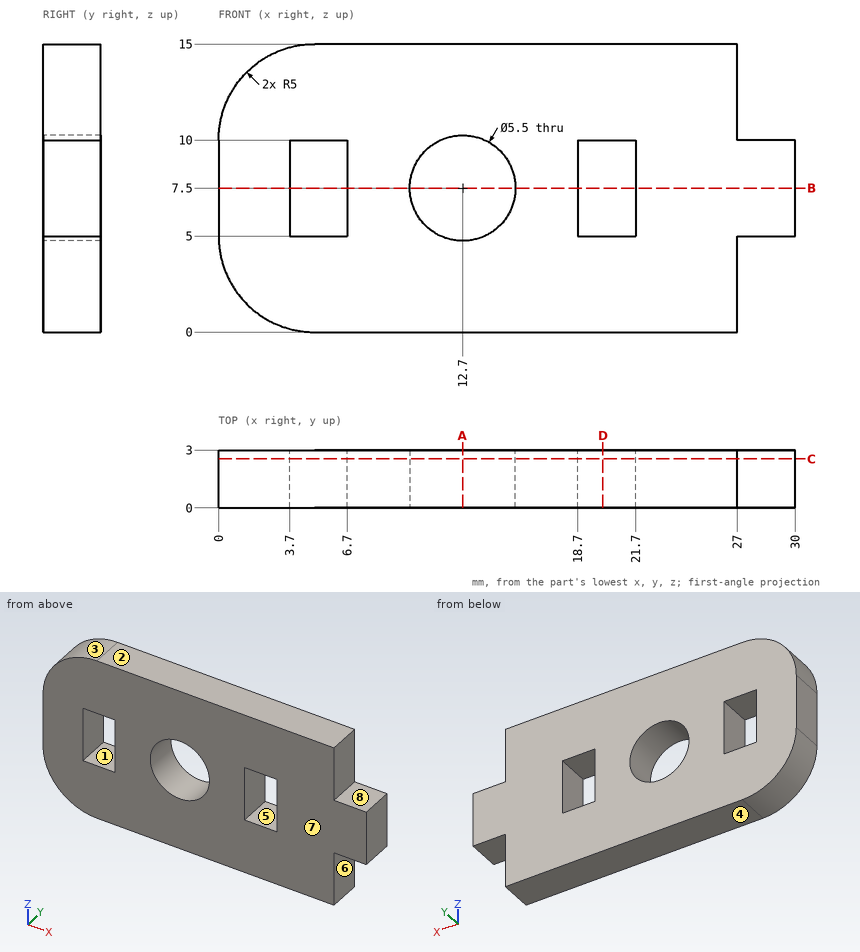
Here's the drawing with two shaded views (mm, measured from the low corner). I have some questions. A direction names the side the tool comes from. Coordinates: 2 decimals unless noted, no trailing zeros. Order: outer loops, then holes, each group sorted by start corner. A loop starts at its lowest first (then second) coordinate and runs counter-clockwise, first axis right, second up. Notation, with made-up numbers: M 25.5,13 L 45.5,13 A29 ccw 45.5,43 Z; hole C -7,81 d6. An arc over 180 degrees is marked long. Answer as CSV lines item,"result".
Item 1: Imagine slicing it at C-C on y = 2.55. Write out the boundary of the cut face in (x, z).
Results found:
outline,"M 0,5 A5 ccw 5,0 L 27,0 L 27,5 L 30,5 L 30,10 L 27,10 L 27,15 L 5,15 A5 ccw 0,10 Z; hole M 3.7,5 L 6.7,5 L 6.7,10 L 3.7,10 Z; hole C 12.7,7.5 d5.5; hole M 18.7,5 L 21.7,5 L 21.7,10 L 18.7,10 Z"
Item 2: Imagine slicing it at B-B on z = 7.5. Write out the boundary of the cut face in (x, y).
Results found:
outline,"M 0,0 L 3.7,0 L 3.7,3 L 0,3 Z; M 6.7,0 L 9.95,0 L 9.95,3 L 6.7,3 Z; M 15.45,0 L 18.7,0 L 18.7,3 L 15.45,3 Z; M 21.7,0 L 30,0 L 30,3 L 21.7,3 Z"
Item 3: Imagine slicing it at D-D on x = 20. Write out the boundary of the cut face in (y, z), plus the area to 3 significant figures.
Results found:
outline,"M 0,0 L 3,0 L 3,5 L 0,5 Z; M 0,10 L 3,10 L 3,15 L 0,15 Z"
area,"30.0 mm2"
Item 4: If I drill on line 1 (X direction, y = 0.9, z = 7.5); line 2 (Z direction, x = 5, y = 2.2); line 3 (X direction, y = 1.9, z = 6.5), over which ranges is the centre line in solid material (lowest first)?
Results found:
line 1,"0 to 3.7, 6.7 to 9.95, 15.45 to 18.7, 21.7 to 30"
line 2,"0 to 5, 10 to 15"
line 3,"0 to 3.7, 6.7 to 10.14, 15.26 to 18.7, 21.7 to 30"
Item 5: We'd pull the mould along X, two halves only. Please class the marked faces 1, 2 and 3: +X half, -X half, draft (parallel to the pull), parting line (faces both ways), or undercut.
Results found:
face 1,"undercut"
face 2,"draft"
face 3,"-X half"
Item 6: On a 3-axis mill with a long thin cutter (end or side, diameter ignored), from which of +Z, -Z, +X, -X, +Y, -Y can I reach the whole of each face in a straight line? I mean the marked faces 4, 5, 6, 7 and 8. Say none if no direction works.
Results found:
face 4,"-Z, +X, -X, +Y, -Y"
face 5,"+Y, -Y"
face 6,"-Z, +X, +Y, -Y"
face 7,"+Z, -Z, +X, -X, -Y"
face 8,"+Z, +X, +Y, -Y"
Item 7: For pin 1 (1.5 mm diameter, centred on y = 1.5, z = 7, fed in from -X); pin 2 (1.5 mm diameter, centred on y = 1.5, z = 2, fed in from +X); pin 3 (3.5 mm diameter, centred on x = 12.7, z = 7.5, fed in from +Y); pin 4 (0.9 mm diameter, centred on x = 28.5, y = 1.5, fed in from -Z), each with a flat end and sliding along its axis, tell me the tip position at first contact or that it passes through.
Results found:
pin 1,"x = 0"
pin 2,"x = 27"
pin 3,"through"
pin 4,"z = 5"
Item 8: Imagine slicing it at A-A on x = 12.7. Write out the boundary of the cut face in (y, z).
Results found:
outline,"M 0,0 L 3,0 L 3,4.75 L 0,4.75 Z; M 0,10.25 L 3,10.25 L 3,15 L 0,15 Z"
